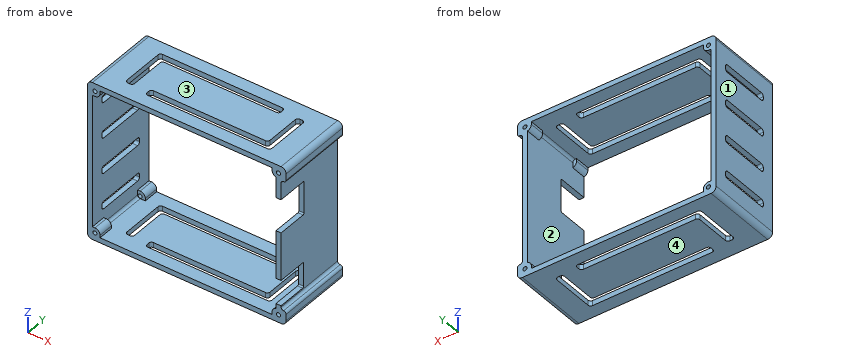
from build123d import *

# Parameters (mm, degrees)
SKETCH4_W             = 72
SKETCH4_H             = 58
BOSS_EXTRUDE3_DEPTH   = 30
SKETCH5_W             = 13.1
SKETCH5_H             = 12.2
SKETCH5_W_2           = 10
SKETCH5_H_2           = 12
CUT_EXTRUDE2_DEPTH    = 13
CUT_EXTRUDE4_REACH    = 91.135
CUT_EXTRUDE3_DEPTH    = 80.649231007
SKETCH21_W            = 3
SKETCH21_H            = 3
SKETCH21_W_2          = 1.5
BOSS_EXTRUDE5_DEPTH   = 6
M2_TAPPED_HOLE1_D     = 1.6
M2_TAPPED_HOLE1_DEPTH = 30
FILLET1_R             = 1
FILLET4_R             = 0.5
FILLET5_R             = 2


# Some blends are built 0.0001 mm under size
with BuildPart() as part:
    # Sketch4 → Boss-Extrude3 (new body)
    with BuildSketch(Plane(origin=(0, 0, 0), x_dir=(1, 0, 0), z_dir=(0, 1, 0))):
        Polygon((-38, -31), (40, -31), (40, -25.5), (38, -25.5), (38, 25.5), (40, 25.5), (40, 31), (-38, 31), align=None)
        Rectangle(SKETCH4_W, SKETCH4_H, mode=Mode.SUBTRACT)
    extrude(amount=BOSS_EXTRUDE3_DEPTH)

    # Sketch5 → Cut-Extrude2 (cut)
    with BuildSketch(Plane(origin=(38, 0, 0), x_dir=(0, 0, -1), z_dir=(1, 0, 0))):
        with Locations((-11.33, 6.1)):
            Rectangle(SKETCH5_W, SKETCH5_H)
        with Locations((19, 6)):
            Rectangle(SKETCH5_W_2, SKETCH5_H_2)
    extrude(amount=-CUT_EXTRUDE2_DEPTH, mode=Mode.SUBTRACT)

    # Sketch15 → Cut-Extrude4 (cut, up to next)
    with BuildSketch(Plane.ZY.offset(38), mode=Mode.PRIVATE) as cut_extrude4_sk1:
        with BuildLine():
            Line((-21.5, 25), (-20.5, 25))
            ThreePointArc((-20.5, 25), (-19.792893219, 24.707106781), (-19.5, 24))
            Line((-19.5, 24), (-19.5, 6))
            ThreePointArc((-19.5, 6), (-19.792893219, 5.292893219), (-20.5, 5))
            Line((-20.5, 5), (-21.5, 5))
            ThreePointArc((-21.5, 5), (-22.207106781, 5.292893219), (-22.5, 6))
            Line((-22.5, 6), (-22.5, 24))
            ThreePointArc((-22.5, 24), (-22.207106781, 24.707106781), (-21.5, 25))
        make_face()
    cut_extrude4_tool1 = extrude(cut_extrude4_sk1.sketch, amount=-CUT_EXTRUDE4_REACH, mode=Mode.PRIVATE) & part.part
    # Sketch15 → Cut-Extrude4 (cut, up to next)
    with BuildSketch(Plane.ZY.offset(38), mode=Mode.PRIVATE) as cut_extrude4_sk2:
        with BuildLine():
            Line((-7.5, 25), (-6.5, 25))
            ThreePointArc((-6.5, 25), (-5.792893219, 24.707106781), (-5.5, 24))
            Line((-5.5, 24), (-5.5, 6))
            ThreePointArc((-5.5, 6), (-5.792893219, 5.292893219), (-6.5, 5))
            Line((-6.5, 5), (-7.5, 5))
            ThreePointArc((-7.5, 5), (-8.207106781, 5.292893219), (-8.5, 6))
            Line((-8.5, 6), (-8.5, 24))
            ThreePointArc((-8.5, 24), (-8.207106781, 24.707106781), (-7.5, 25))
        make_face()
    cut_extrude4_tool2 = extrude(cut_extrude4_sk2.sketch, amount=-CUT_EXTRUDE4_REACH, mode=Mode.PRIVATE) & part.part
    cut_extrude4_1 = cut_extrude4_tool1.solids().sort_by_distance((-38, 15, -21))[0]
    add(cut_extrude4_1, mode=Mode.SUBTRACT)
    cut_extrude4_2 = cut_extrude4_tool2.solids().sort_by_distance((-38, 15, -7))[0]
    add(cut_extrude4_2, mode=Mode.SUBTRACT)
    cut_extrude4 = cut_extrude4_1 + cut_extrude4_2  # Cut-Extrude4 as one shape, for the pattern or mirror that repeats it

    # Mirror1: Cut-Extrude4 across plane
    add(cut_extrude4.mirror(Plane.XY), mode=Mode.SUBTRACT)

    # Sketch14 → Cut-Extrude3 (cut, through all)
    with BuildSketch(Plane.XY.offset(-31)):
        with BuildLine():
            Line((-28, 7.5), (-28, 24))
            ThreePointArc((-28, 24), (-27.707106781, 24.707106781), (-27, 25))
            Line((-27, 25), (20, 25))
            ThreePointArc((20, 25), (20.707106781, 24.707106781), (21, 24))
            Line((21, 24), (21, 23))
            ThreePointArc((21, 23), (20.707106781, 22.292893219), (20, 22))
            Line((20, 22), (-24, 22))
            ThreePointArc((-24, 22), (-24.707106781, 21.707106781), (-25, 21))
            Line((-25, 21), (-25, 7.5))
            ThreePointArc((-25, 7.5), (-25.292893219, 6.792893219), (-26, 6.5))
            Line((-26, 6.5), (-27, 6.5))
            ThreePointArc((-27, 6.5), (-27.707106781, 6.792893219), (-28, 7.5))
        make_face()
        with BuildLine():
            Line((27, 22.5), (27, 9))
            ThreePointArc((27, 9), (26.707106781, 8.292893219), (26, 8))
            Line((26, 8), (-18, 8))
            ThreePointArc((-18, 8), (-18.707106781, 7.707106781), (-19, 7))
            Line((-19, 7), (-19, 6))
            ThreePointArc((-19, 6), (-18.707106781, 5.292893219), (-18, 5))
            Line((-18, 5), (29, 5))
            ThreePointArc((29, 5), (29.707106781, 5.292893219), (30, 6))
            Line((30, 6), (30, 22.5))
            ThreePointArc((30, 22.5), (29.707106781, 23.207106781), (29, 23.5))
            Line((29, 23.5), (28, 23.5))
            ThreePointArc((28, 23.5), (27.292893219, 23.207106781), (27, 22.5))
        make_face()
    extrude(amount=CUT_EXTRUDE3_DEPTH, mode=Mode.SUBTRACT)

    # Sketch21 → Boss-Extrude5 (add)
    with BuildSketch(Plane.XZ):
        with Locations((-34.5, 27.5)):
            Rectangle(SKETCH21_W, SKETCH21_H)
        with Locations((35.25, 27.5)):
            Rectangle(SKETCH21_W_2, SKETCH21_H)
        with Locations((35.25, -27.5)):
            Rectangle(SKETCH21_W_2, SKETCH21_H)
        with Locations((-34.5, -27.5)):
            Rectangle(SKETCH21_W, SKETCH21_H)
    boss_extrude5 = extrude(amount=-BOSS_EXTRUDE5_DEPTH)

    # M2 Tapped Hole1
    with Locations(Plane(origin=(0, 0, 0), x_dir=(-1, 0, 0), z_dir=(0, -1, 0))):
        with Locations((35, 28), (35, -28), (-37, -28), (-37, 28)):
            m2_tapped_hole1 = Hole(M2_TAPPED_HOLE1_D / 2, depth=M2_TAPPED_HOLE1_DEPTH)

    # Fillet1
    fillet1_edges = [part.edges().sort_by_distance(p)[0] for p in [
        (-36, 18, 29),
        (-36, 18, -29),
        (36, 18, 29),
        (36, 18, -29),
        (40, 15, -25.5),
        (38, 15, -25.5),
        (38, 15, 25.5),
        (40, 15, 25.5),
    ]]
    fillet(fillet1_edges, radius=FILLET1_R - 0.0001)  # a hair under: the kernel refuses the full size

    # Fillet4
    fillet4_edges = [part.edges().sort_by_distance(p)[0] for p in [
        (37, 12.2, 4.78),
        (37, 12.2, 17.88),
        (37, 12, -24),
        (37, 12, -14),
    ]]
    fillet(fillet4_edges, radius=FILLET4_R)

    # Mirror2: Boss-Extrude5, M2 Tapped Hole1 across plane
    add(boss_extrude5.mirror(Plane(origin=(0, 15, 0), x_dir=(0, 0, 1), z_dir=(0, -1, 0))))
    add(m2_tapped_hole1.mirror(Plane(origin=(0, 15, 0), x_dir=(0, 0, 1), z_dir=(0, -1, 0))), mode=Mode.SUBTRACT)

    # Fillet5
    # the kernel refuses this fillet: 2 mm, written as the material it takes off along each edge
    with BuildSketch(Plane(origin=(40, -5, 31), x_dir=(-1, 0, 0), z_dir=(0, 1, 0)), Plane(origin=(-38, -5, 31), x_dir=(0, 0, -1), z_dir=(0, 1, 0)), Plane(origin=(-38, -5, -31), x_dir=(1, 0, 0), z_dir=(0, 1, 0)), Plane(origin=(40, -5, -31), x_dir=(0, 0, 1), z_dir=(0, 1, 0))) as fillet5_piece_1:
        with BuildLine():
            CenterArc((FILLET5_R, -FILLET5_R), FILLET5_R, 90, 90)
            Line((0, -FILLET5_R), (-FILLET5_R * 0.02, -FILLET5_R))
            Line((-FILLET5_R * 0.02, -FILLET5_R), (-FILLET5_R * 0.02, FILLET5_R * 0.02))
            Line((-FILLET5_R * 0.02, FILLET5_R * 0.02), (FILLET5_R, FILLET5_R * 0.02))
            Line((FILLET5_R, FILLET5_R * 0.02), (FILLET5_R, 0))
        make_face()
    extrude(amount=40, mode=Mode.SUBTRACT)
    with BuildSketch(Plane(origin=(-33, -5, 26), x_dir=(-1, 0, 0), z_dir=(0, 1, 0)), Plane(origin=(-33, -5, -26), x_dir=(0, 0, -1), z_dir=(0, 1, 0)), Plane(origin=(-33, 35, -26), x_dir=(-1, 0, 0), z_dir=(0, -1, 0))) as fillet5_piece_2:
        with BuildLine():
            CenterArc((FILLET5_R, FILLET5_R), FILLET5_R, 180, 90)
            Line((0, FILLET5_R), (-FILLET5_R * 0.02, FILLET5_R))
            Line((-FILLET5_R * 0.02, FILLET5_R), (-FILLET5_R * 0.02, -FILLET5_R * 0.02))
            Line((-FILLET5_R * 0.02, -FILLET5_R * 0.02), (FILLET5_R, -FILLET5_R * 0.02))
            Line((FILLET5_R, -FILLET5_R * 0.02), (FILLET5_R, 0))
        make_face()
    extrude(amount=16, mode=Mode.SUBTRACT)
    with BuildSketch(Plane(origin=(34.5, -4.841229183, 26), x_dir=(1, 0, 0), z_dir=(0, 1, 0))) as fillet5_piece_3:
        with BuildLine():
            CenterArc((2, -1.936491673), FILLET5_R, 104.477512186, 75.522487814)
            Line((0, -1.936491673), (-0.04, -1.936491673))
            Line((-0.04, -1.936491673), (-0.04, 0))
            Line((-0.04, 0), (0, 0.04))
            ThreePointArc((0, 0.04), (0.75, 0.04), (1.49, 0.038729833))
            Line((1.49, 0.038729833), (1.5, 0))
        make_face()
    extrude(amount=15.682458366, mode=Mode.SUBTRACT)
    with BuildSketch(Plane(origin=(34.5, -4.841229183, -26), x_dir=(1, 0, 0), z_dir=(0, 1, 0))) as fillet5_piece_4:
        with BuildLine():
            CenterArc((2, 1.936491673), FILLET5_R, 180, 75.522487814)
            Line((0, 1.936491673), (-0.04, 1.936491673))
            Line((-0.04, 1.936491673), (-0.04, 0))
            Line((-0.04, 0), (0, -0.04))
            ThreePointArc((0, -0.04), (0.75, -0.04), (1.49, -0.038729833))
            Line((1.49, -0.038729833), (1.5, 0))
        make_face()
    extrude(amount=15.682458366, mode=Mode.SUBTRACT)
    with BuildSketch(Plane(origin=(-33, 35, 26), x_dir=(-1, 0, 0), z_dir=(0, -1, 0))) as fillet5_piece_5:
        with BuildLine():
            CenterArc((FILLET5_R, -FILLET5_R), FILLET5_R, 90, 90)
            Line((0, -FILLET5_R), (-FILLET5_R * 0.02, -FILLET5_R))
            Line((-FILLET5_R * 0.02, -FILLET5_R), (-FILLET5_R * 0.02, FILLET5_R * 0.02))
            Line((-FILLET5_R * 0.02, FILLET5_R * 0.02), (FILLET5_R, FILLET5_R * 0.02))
            Line((FILLET5_R, FILLET5_R * 0.02), (FILLET5_R, 0))
        make_face()
    extrude(amount=16, mode=Mode.SUBTRACT)
    with BuildSketch(Plane(origin=(34.5, 34.841229183, 26), x_dir=(0, 0, 1), z_dir=(0, -1, 0))) as fillet5_piece_6:
        with BuildLine():
            CenterArc((1.936491673, -2), FILLET5_R, 90, 75.522487814)
            Line((0, -1.5), (-0.038729833, -1.49))
            ThreePointArc((-0.038729833, -1.49), (-0.04, -0.75), (-0.04, 0))
            Line((-0.04, 0), (0, 0.04))
            Line((0, 0.04), (1.936491673, 0.04))
            Line((1.936491673, 0.04), (1.936491673, 0))
        make_face()
    extrude(amount=15.682458366, mode=Mode.SUBTRACT)
    with BuildSketch(Plane(origin=(34.5, 34.841229183, -26), x_dir=(0, 0, -1), z_dir=(0, -1, 0))) as fillet5_piece_7:
        with BuildLine():
            CenterArc((1.936491673, 2), FILLET5_R, 194.477512186, 75.522487814)
            Line((0, 1.5), (-0.038729833, 1.49))
            ThreePointArc((-0.038729833, 1.49), (-0.04, 0.75), (-0.04, 0))
            Line((-0.04, 0), (0, -0.04))
            Line((0, -0.04), (1.936491673, -0.04))
            Line((1.936491673, -0.04), (1.936491673, 0))
        make_face()
    extrude(amount=15.682458366, mode=Mode.SUBTRACT)


solid = part.part
Model file for the job. Use its own axes, mm. Face numbers are marked on the shaded views. Give positions to 0.01 mm unless a question says otherwise; leave off trailing zeros. Loops run counter-clockwise (first coordinate to the right, second up) from the corner with the lowest first, then second, coordinate; pieces in that order, holes last.
1) Saw through at C-C (y = 27). Count the separate pieces of the cut face and the enclosed holes in it, plus the area to 3 significant figures.
2) Flat gauge pin, fed straight in: pin 1 Ø6 at (y, z) = (15, -22) entering from +X. Where does the tip first touch, or does it go through?
3) Pull direction Z, two halves, no side cores. Call the marked faces 1, 2, 3 and 4: +Z half, -Z half, draft (parallel to the pull), parting line (faces both ways), or undercut.
4) Saw through at A-A (z = -18). Write the cut outline in (x, y), plus the area to 3 significant figures.
5) Wall check: line 1 (Z direction, x = 37, y = 15); line 2 (X direction, y = 3.05, z = 28); line 3 (Z direction, x = -35, y = 2.1). Give the ranges that are in metal, low to high.
6) Saw through at B-B (x = 15.5). Write the cut outline in (y, z), plus the area to 3 significant figures.
Answer block:
1. separate pieces: 1
1. enclosed holes: 5
1. area: 570 mm2
2. pin 1: stops at x = 38.13
3. face 1: draft
3. face 2: undercut
3. face 3: +Z half
3. face 4: -Z half
4. outline: (-38, 0) - (-36, 0) - (-36, 30) - (-38, 30) - close; (36, 12) - (38, 12) - (38, 30) - (36, 30) - close
4. area: 96.0 mm2
5. line 1: z = -31 to -28.8, -27.2 to 27.2, 28.8 to 31
5. line 2: x = -38 to -35.8, -34.2 to -33, 34.5 to 36.2, 37.8 to 40
5. line 3: z = -31 to -28.8, -27.2 to -26, 26 to 27.2, 28.8 to 31
6. outline: (0, -31) - (5, -31) - (5, -29) - (0, -29) - close; (0, 29) - (5, 29) - (5, 31) - (0, 31) - close; (8, -31) - (22, -31) - (22, -29) - (8, -29) - close; (8, 29) - (22, 29) - (22, 31) - (8, 31) - close; (25, -31) - (30, -31) - (30, -29) - (25, -29) - close; (25, 29) - (30, 29) - (30, 31) - (25, 31) - close
6. area: 96.0 mm2
